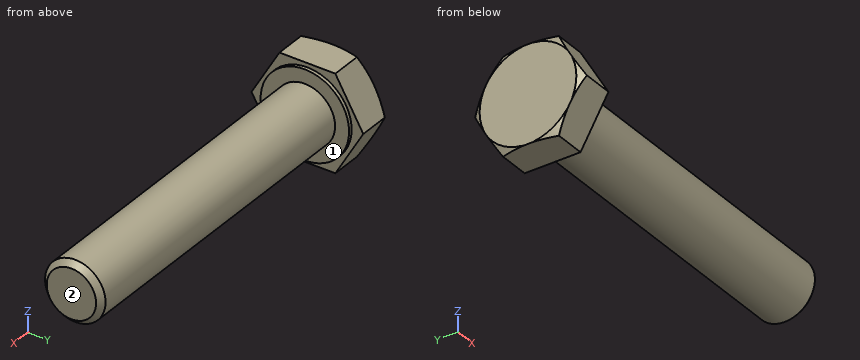
Autodesk Inventor part; units mm, degrees
ref_plane "Work Plane1" through (1.525, 0, 0) normal (0, 0, 1) x (1, 0, 0)
ref_plane "YZ Plane" through (0, 0, 0) normal (1, 0, 0) x (0, 1, 0)
ref_plane "XZ Plane" through (0, 0, 0) normal (0, 1, 0) x (-1, 0, 0)
sketch "Skizze1" plane through (0, 0, 0) normal (0, 0, 1) x (1, 0, 0)
  line L0 (0, 7.315) -> (0, 5)
  line L1 (29, 5) -> (55, 5)
  line L2 (55, 5) -> (55, 0)
  line L3 (55, 0) -> (-0.6001, 0)
  line L4 (-11.7201, 0) -> (66.12, 0)
  line L5 (-0.6001, 0) -> (-0.6001, 7.315)
  line L6 (-0.6001, 7.315) -> (0, 7.315)
  line L7 (29, 5) -> (28.0797, 5)
  line L8 (28.0797, 5) -> (0, 5)
  line L9 (0, -1.463) -> (0, 8.778)
  dimension "d0" = 55
  dimension "d1" = 26
  dimension "d2" = 10
  dimension "d9" = 0.6001
  dimension "d10" = 14.63
  dimension "d13" = 0.9203
  dimension "d14" = 10
revolve "Körper" add sketch "Skizze1" angle 360 about axis through (55, 0, 0) along (-1, 0, 0)
sketch "Skizze2" plane through (-0.6001, 0, 0) normal (-1, 0, 0) x (0, 0, 1)
  line L0 (0, 9.2376) -> (8, 4.6188)
  line L1 (8, 4.6188) -> (8, -4.6188)
  line L2 (8, -4.6188) -> (0, -9.2376)
  line L3 (0, -9.2376) -> (-8, -4.6188)
  line L4 (-8, -4.6188) -> (-8, 4.6188)
  line L5 (-8, 4.6188) -> (0, 9.2376)
  point P0 (0, 0)
  point P1 (0, 0)
  dimension "d11" = 16
extrude "Kopf" add sketch "Skizze2" along normal blind 5.8
sketch "Skizze4" plane through (0, 0, 0) normal (0, 0, 1) x (1, 0, 0)
  line L0 (-6.4001, 8) -> (-6.4001, 9.2376)
  line L1 (-6.4001, 9.2376) -> (-5.6856, 9.2376)
  line L2 (-5.6856, 9.2376) -> (-6.4001, 8)
  line L3 (-7.5601, 0) -> (0.5599, 0)
  line L4 (-0.6001, 9.2376) -> (-6.4001, 9.2376)
  line L5 (-6.4001, 4.6188) -> (-6.4001, 9.2376)
  dimension "d5" = 30
  dimension "d19" = 16
revolve "Fase1" cut sketch "Skizze4" angle 360 about axis through (-10, 0, 0) along (1, 0, 0)
thread "Gewinde"
chamfer "Fase2" distance 0.9202 distance2 0.9203 1 edges at (55, -5, 0) measured on face at (55, 1.2281, 0.495)
ref_plane "Work Plane1" through (1.525, 0, 0) normal (0, 0, 1) x (1, 0, 0)
equation "\"d0\" = NLG"
equation "\"d1\" = GEL"
equation "\"d2\" = GD"
equation "\"d10\" = SD2"
equation "\"d14\" = BDM"
equation "\"d11\" = SW"
equation "\"d3\" = KOH - SD"
equation "\"d5\" = ANG1"
equation "\"d19\" = SW0"
equation "\"d15\" = GEL"
equation "\"d6\" = -0.5 * SPD + 0.5 * GD"
equation "\"NLG\" = 55"
equation "\"GD\" = NND"
equation "\"BDM\" = NND"
equation "\"KOH\" = 6.4"
equation "\"GEL\" = 26"
equation "\"SW\" = 16"
equation "\"SW0\" = SW"
equation "\"SPD\" = NND - 1.2269 * PTC"
equation "\"SD2\" = 14.63"
equation "\"SD\" = 0.6"
equation "\"ANG1\" = 30deg"
equation "\"GAL\" = 0.61345 * PTC"
equation "\"GUL\" = 0.61345 * PTC"
equation "\"RR\" = 0.4"
equation "\"GD1\" = THREADDIA - 1.2269 * PTC"
equation "\"SDH\" = SD2"
equation "\"TOA\" = 30deg"
equation "\"PTC\" = 1.5"
equation "\"E0\" = 1.155 * SW"
properties part number "ISO 4014 - M10 x 55" material "Edelstahl, 440C"
The model under review builds one solid part; all positions refer to its coordinate system, in mm. Face numbers are marked on the shaded views. A direction names the side the tool comes from. Coordinates: 2 decimals unless noted, no trailing zeros. Loops run counter-clockwise (first coordinate to the right, second up) from the corner with the lowest first, then second, coordinate; pieces in that order, holes last. Notation, with made-up numbers: M 24,7.5 L 81,7.5 A29 cw 81,33.5 Z; hole C 50,39.5 d2. An arc over 180 degrees is marked long. Put each result on its own line as item: value. Start each with the question number.
Q1. Add section A-A (x = 47). Write out the cut boundary in (y, z).
Q2. For the marked faces 1 and 2, list the 3-axis set-ups (+Z, -Z, +X, -X, +Y, -Y) from which the entire face can be reached by the end or side of a thin tool; tool diameter is ignored.
Q3. Wall thickness on line 1 (Z direction, x = 47.5, y = 3); line 2 (X direction, y = 3.5, z = 4); line 3 (X direction, y = 6.5, z = 3.5): over which ranges is each line inside the solid? List them lowest first.
Q4. Clearance check with flat-ended pins moving along their axes: pin 1 (1 mm diameter, centred on x = 48.5, y = -1.5, fed in from +Z); pin 2 (1.5 mm diameter, centred on y = 1.5, z = -6, fed in from +X); pin 3 (2 mm diameter, centred on x = 0.5, y = 0, fed in from -Z) (3 decimals). State where each tip first meets the part, or that it passes through.
Answers:
1. outline: C 0,0 d10
2. face 1: +X
2. face 2: +Z, -Z, +X, +Y, -Y
3. line 1: z = -4 to 4
3. line 2: x = -6.4 to 0
3. line 3: x = -6.4 to -0.6
4. pin 1: stops at z = 4.9
4. pin 2: stops at x = 0
4. pin 3: stops at z = -7.315
